Here's how the part is built. I have some questions about the finished solid (model axes, mm). Face numbers are marked on the shaded views. A direction names the side the tool comes from. Give positions to 0.01 mm unless a question says otherwise; leave off trailing zeros. Loops run counter-clockwise (first coordinate to the right, second up) from the corner with the lowest first, then second, coordinate; pieces in that order, holes last.
Q1. I need wall thicknesses on line 1 (Z direction, x = -17, y = 11); line 2 (Z direction, x = -20, y = 3.25); line 3 (X direction, y = 18.5, z = 6). Which ranges of each line are inside material? Lowest first, please.
Q2. If we section it at A-A (z = 0): Please give me the cut outline in (x, y) (3 decimals).
Q3. If we section it at B-B (y = 10.5): Please give me the cut outline in (x, z) (3 decimals), plus the area to 3 significant figures.
Q4. For the marked faces 1, 2, 3 and 4, which set-ups out of +Z, -Z, +X, -X, +Y, -Y let a thin tool reach every point of the face, with its end or its side?
Q5. We'd pull the mould along Z, two halves only. Please class the marked faces 5, 6 and 7: +Z half, -Z half, draft (parallel to the pull), parting line (faces both ways), or undercut.
Q6. If we section it at C-C (z = 5.5): Please give me the cut outline in (x, y), plus the area to 3 significant figures.
Q7. Will these pins go through, and if not, where does the flat tip stop? P1, Ø4, axis at y = 12.5, z = -7.5, coming from the -X side; P2, Ø1, axis at x = -18, y = 3.5, coming from the +Z side; P3, Ø2.5, axis at x = -18, y = 7, coming from the -Z side; P4, Ø2, axis at x = -19.125, z = 0, coming from the -Y side.
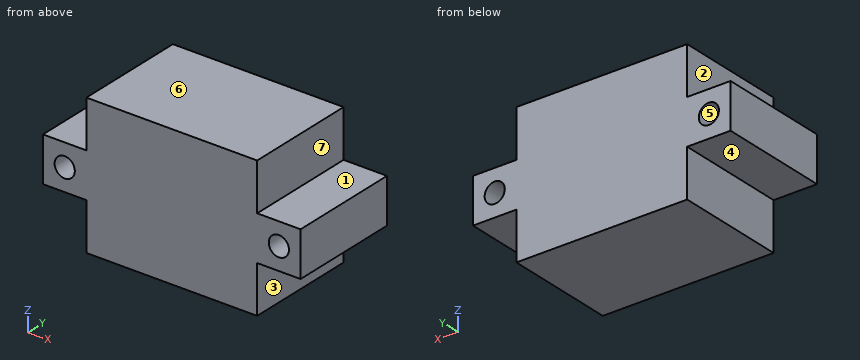
from build123d import *

# Parameters (mm, degrees)
BOSS_EXTRU_1_DEPTH = 20
D_GAGEMENT_M31_D   = 3.6


with BuildPart() as part:
    # Esquisse1 → Boss.-Extru.1 (new body)
    with BuildSketch(Plane(origin=(0, 0, 0), x_dir=(1, 0, 0), z_dir=(0, 1, 0))):
        Polygon((-15.25, -12.5), (15.25, -12.5), (15.25, -4.001343409), (23, -4.001343409), (23, 4.001343409), (15.25, 4.001343409), (15.25, 12.5), (-15.25, 12.5), (-15.25, 4.001343409), (-23, 4.001343409), (-23, -4.001343409), (-15.25, -4.001343409), align=None)
    extrude(amount=BOSS_EXTRU_1_DEPTH)

    # Dégagement M31 (through all)
    with Locations(Plane(origin=(0, 20, 0), x_dir=(1, 0, 0), z_dir=(0, 1, 0))):
        with Locations((-19.125, 0), (19.125, 0)):
            Hole(D_GAGEMENT_M31_D / 2)


solid = part.part
Check sheet entries:
1. line 1: z = -4 to 4
1. line 2: z = -4 to -1.57, 1.57 to 4
1. line 3: x = -15.25 to 15.25
2. outline: (-23, 0) - (-20.925, 0) - (-20.925, 20) - (-23, 20) - close; (-17.325, 0) - (17.325, 0) - (17.325, 20) - (-17.325, 20) - close; (20.925, 0) - (23, 0) - (23, 20) - (20.925, 20) - close
3. outline: (-23, -4.001) - (-15.25, -4.001) - (-15.25, -12.5) - (15.25, -12.5) - (15.25, -4.001) - (23, -4.001) - (23, 4.001) - (15.25, 4.001) - (15.25, 12.5) - (-15.25, 12.5) - (-15.25, 4.001) - (-23, 4.001) - close; hole circle Ø3.6 at (-19.125, 0); hole circle Ø3.6 at (19.125, 0)
3. area: 866 mm2
4. face 1: +Z, +X, +Y, -Y
4. face 2: +Z, -X, +Y, -Y
4. face 3: -Z, +X, +Y, -Y
4. face 4: -Z, -X, +Y, -Y
5. face 5: undercut
5. face 6: +Z half
5. face 7: draft
6. outline: (-15.25, 0) - (15.25, 0) - (15.25, 20) - (-15.25, 20) - close
6. area: 610 mm2
7. P1: stops at x = -15.25
7. P2: stops at z = 4
7. P3: stops at z = -4
7. P4: passes through
